```python
from build123d import *

# Parameters (mm, degrees)
SZKIC1_R                    = 14.3
DODANIE_WYCI_GNI_CIE1_DEPTH = 12.96
WYTNIJ_WYCI_GNI_CIE1_REACH  = 14.96
SZKIC2_R                    = 8.4
SZKIC3_R                    = 9.42
WYTNIJ_WYCI_GNI_CIE2_DEPTH  = 1.18
SZKIC5_R                    = 10.19
WYTNIJ_WYCI_GNI_CIE3_DEPTH  = 1.38


with BuildPart() as part:
    # Szkic1 → Dodanie-wyciągnięcie1 (new body)
    with BuildSketch(Plane.XY):
        Circle(SZKIC1_R)
    extrude(amount=DODANIE_WYCI_GNI_CIE1_DEPTH)

    # Szkic2 → Wytnij-wyciągnięcie1 (cut, up to next)
    with BuildSketch(Plane.XY.offset(12.96), mode=Mode.PRIVATE) as wytnij_wyci_gni_cie1_sk1:
        Circle(SZKIC2_R)
    wytnij_wyci_gni_cie1_tool1 = extrude(wytnij_wyci_gni_cie1_sk1.sketch, amount=-WYTNIJ_WYCI_GNI_CIE1_REACH, mode=Mode.PRIVATE) & part.part
    add(wytnij_wyci_gni_cie1_tool1.solids().sort_by_distance((0, 0, 12.96))[0], mode=Mode.SUBTRACT)

    # Szkic3 → Wytnij-wyciągnięcie2 (cut)
    with BuildSketch(Plane.XY.offset(12.96)):
        Circle(SZKIC3_R)
    wytnij_wyci_gni_cie2 = extrude(amount=-WYTNIJ_WYCI_GNI_CIE2_DEPTH, mode=Mode.SUBTRACT)

    # Lustro1: Wytnij-wyciągnięcie2 across plane
    add(wytnij_wyci_gni_cie2.mirror(Plane.XY.offset(6.48)), mode=Mode.SUBTRACT)

    # Szkic5 → Wytnij-wyciągnięcie3 (cut, symmetric)
    with BuildSketch(Plane.XY.offset(6.48)):
        Circle(SZKIC5_R)
    extrude(amount=WYTNIJ_WYCI_GNI_CIE3_DEPTH, both=True, mode=Mode.SUBTRACT)


solid = part.part
```
Design review of the part built by this model. Coordinates are the model's own, in mm. A direction names the side the tool comes from. Give positions to 0.01 mm unless a question says otherwise; leave off trailing zeros. Write each loop counter-clockwise with the first axis right and the second up, starting at its lowest first coordinate (ties: lowest second). Pieces come first, ordered by that corner, then holes.
(1) Mouldability with a two-part tool opening along Y and no side actions: class faces 1 (the face through (9.3, -3, 0)), 2 (the face through (-2.209, -9.948, 6.499)), 3 (the face through (-1.86, 14.18, 6.39)) as +Y half, -Y half, draft (parallel to the pull), parting line (faces both ways), or undercut.
Checked values:
face 1: draft
face 2: undercut
face 3: parting line
(2) Clearance check with flat-ended pins moving along their axes: pin 1 Ø12 at (x, y) = (0, 0) entering from +Z; pin 2 Ø17 at (x, y) = (0, 0) entering from -Z; pin 3 Ø4 at (x, z) = (-6, 2) entering from -Y; pin 4 Ø1.5 at (y, z) = (-11, 3.5) entering from -X. State where each tip first meets the part, or that it passes through.
Checked values:
pin 1: passes through
pin 2: stops at z = 1.18
pin 3: stops at y = -13.73
pin 4: stops at x = -9.97
(3) Add section C-C (z = 9.75). Give the boundary of the cut face in (x, y), and give its area (3 significant figures).
Checked values:
outline: circle Ø28.6 at (0, 0); hole circle Ø16.8 at (0, 0)
area: 421 mm2
(4) Tool access review of faces 4 (the face through (-2.042, -9.196, 0.582)), 5 (the face through (-2.042, -9.196, 12.378)), 6 (the face through (-4, 8, 7.86)), 7 (the face through (9.3, -3, 12.96)): name each direction out of +Z, -Z, +X, -X, +Y, -Y from which nothing blocks a thin tool from reaching the whole face with its end or side.
Checked values:
face 4: -Z
face 5: +Z
face 6: none
face 7: +Z, +X, -X, +Y, -Y
(5) Add section D-D (y = 11). Give the boundary of the cut face in (x, z).
Checked values:
outline: (-9.14, 0) - (9.14, 0) - (9.14, 12.96) - (-9.14, 12.96) - close
(6) Wall thickness on line 1 along Y through (x, z) = (0, 6); line 2 along Y through (x, z) = (0, 12.4); line 3 along Z through (x, y) = (0, 10): over which ranges is each line inside the solid? List them lowest first.
Checked values:
line 1: y = -14.3 to -10.19, 10.19 to 14.3
line 2: y = -14.3 to -9.42, 9.42 to 14.3
line 3: z = 0 to 5.1, 7.86 to 12.96
(7) Add section A-A (y = 0). Give the boundary of the cut face in (x, z), and give its area (3 significant figures).
Checked values:
outline: (-14.3, 0) - (-9.42, 0) - (-9.42, 1.18) - (-8.4, 1.18) - (-8.4, 5.1) - (-10.19, 5.1) - (-10.19, 7.86) - (-8.4, 7.86) - (-8.4, 11.78) - (-9.42, 11.78) - (-9.42, 12.96) - (-14.3, 12.96) - close; (8.4, 1.18) - (9.42, 1.18) - (9.42, 0) - (14.3, 0) - (14.3, 12.96) - (9.42, 12.96) - (9.42, 11.78) - (8.4, 11.78) - (8.4, 7.86) - (10.19, 7.86) - (10.19, 5.1) - (8.4, 5.1) - close
area: 138 mm2
